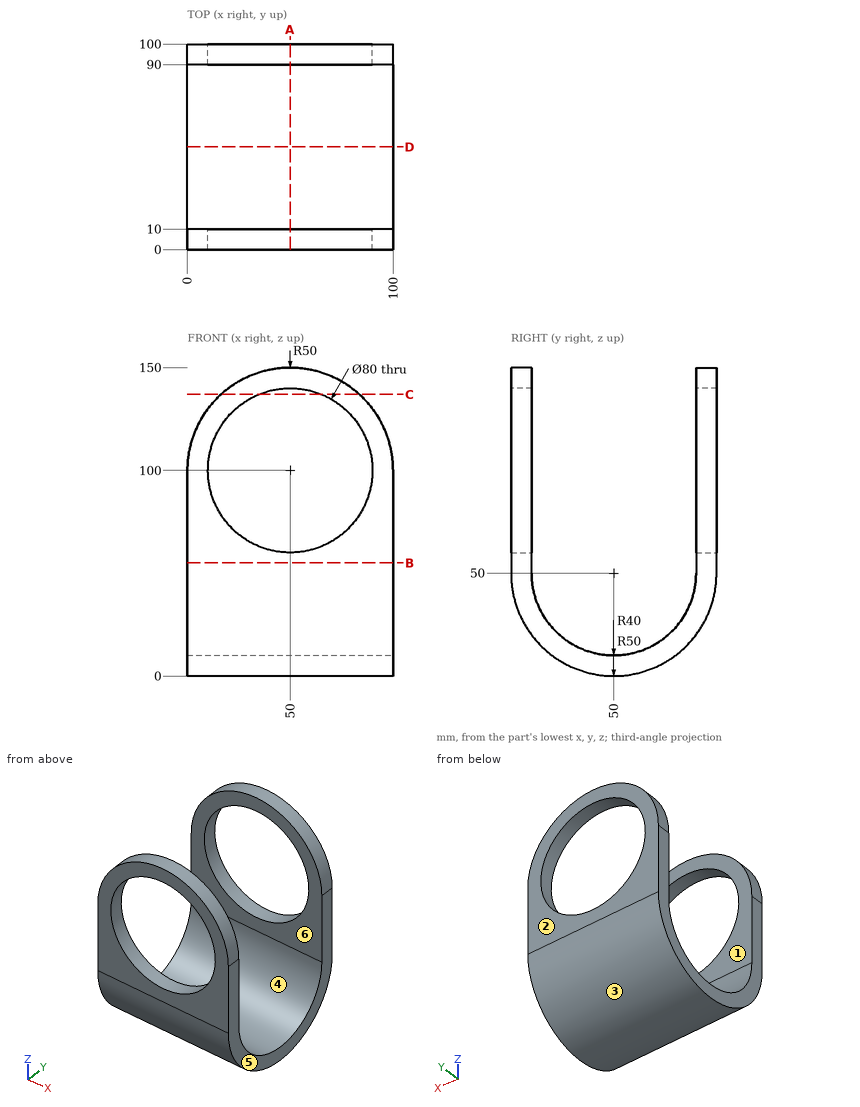
Check sheet for the drawn part. Datum: minimum x, y, z corner. Units: mm. A direction names the side the tool comes from. Round coordinates to 2 decimals unless told otherwise and drop trailing zeros. Order: outer loops, then holes, each group sorted by start corner. A loop starts at its lowest first (then second) coordinate and runs counter-clockwise, first axis right, second up. Notation, with made-up numbers: (65.5, -39) -> (103.5, -39) arc R21 ccw to (103.5, -12) -> close; hole circle Ø6 at (75.5, 13). An arc over 180 degrees is marked (long way). Return JSON: item names as keys, results as strings. Group by question number.
Q1. Section check C-C, the plane z = 137. Record the boundary of the cut face in (x, y).
Q2. Section check A-A, the plane x = 50. Record the boundary of the cut face in (y, z).
Q3. Material ranges on probe 1 along X at (y, z) = (92, 100); probe 2 along Z at (x, y) = (51.5, 95.5), recorded low to high. Write a range as from..to.
Q4. Release check for a two-part mould opening along Y. For the marked faces 1, 2, 3 and 4 record: released by +Y, released by -Y, zero draft, split by the parting line, or undercut.
Q5. Section check B-B, the plane z = 55. Record the boundary of the cut face in (x, y), plus the area to 3 significant figures.
Q6. Section check D-D, the plane y = 50. Record the boundary of the cut face in (x, z), plus the area to 3 significant figures.
Q7. Gauge pin test, flat ends, axial feed: pin 1 (3 mm diameter, centred on x = 70.5, y = 83, fed in from -Z); pin 2 (12 mm diameter, centred on x = 37, z = 75, fed in from +Y); pin 3 (2 mm diameter, centred on x = 33.5, y = 44, fed in from +Z); pin 4 (12 mm diameter, centred on x = 25.5, z = 49, fed in from +Y). Record the tip position at first contact, or that the pin passes through.
Q8. Tool access check on the marked faces 5 and 6. Record the directions out of +Z, -Z, +X, -X, +Y, -Y that give a thin tool (end or side, any length) a straight path to the whole face; none if there is none.
Numbers:
{
 "1": {"outline": "(16.37, 0) -> (34.8, 0) -> (34.8, 10) -> (16.37, 10) -> close; (16.37, 90) -> (34.8, 90) -> (34.8, 100) -> (16.37, 100) -> close; (65.2, 0) -> (83.63, 0) -> (83.63, 10) -> (65.2, 10) -> close; (65.2, 90) -> (83.63, 90) -> (83.63, 100) -> (65.2, 100) -> close"},
 "2": {"outline": "(0, 50) arc R50 ccw to (100, 50) -> (100, 60) -> (90, 60) -> (90, 50) arc R40 cw to (10, 50) -> (10, 60) -> (0, 60) -> close; (0, 140) -> (10, 140) -> (10, 150) -> (0, 150) -> close; (90, 140) -> (100, 140) -> (100, 150) -> (90, 150) -> close"},
 "3": {"probe 1": "0..10, 90..100", "probe 2": "29.27..60.03, 139.97..149.98"},
 "4": {"face 1": "undercut", "face 2": "released by +Y", "face 3": "split by the parting line", "face 4": "undercut"},
 "5": {"outline": "(0, 0) -> (100, 0) -> (100, 10) -> (0, 10) -> close; (0, 90) -> (100, 90) -> (100, 100) -> (0, 100) -> close", "area": "2,000 mm^2"},
 "6": {"outline": "(0, 0) -> (100, 0) -> (100, 10) -> (0, 10) -> close", "area": "1,000 mm^2"},
 "7": {"pin 1": "z = 11.17", "pin 2": "through", "pin 3": "z = 10.62", "pin 4": "y = 100"},
 "8": {"face 5": "+Z, -Z, +X, +Y, -Y", "face 6": "+Z, +X, -X"}
}
